The model under review builds one solid part; all positions refer to its coordinate system, in mm. A direction names the side the tool comes from. Round coordinates to 2 decimals unless told otherwise and drop trailing zeros.
Item 1: Machinability: for faces 4 (the face through (-21.863, -2.882, -0.063)), 5 (the face through (2.794, -1, 0)), 6 (the face through (-48.549, -0.705, -0.04)), 7 (the face through (0, 1, 0)), which of the approach directions +Z, -Z, +X, -X, +Y, -Y give a long, thin tool a straight path to every point of the face, cutting with its end or side? Answer none if there is none.
Item 2: Draft analysis for pull direction X (two halves, no side actions). For faces 1 (the face through (-0.387, 1.841, -0.04)), 2 (the face through (-48.661, 0.744, -0.04)), 3 (the face through (-22.638, 2.882, -0.063)), state which applies: +X half, -X half, draft (parallel to the pull), parting line (faces both ways), or undercut.
Item 3: To check wall thickness, follow L1, parallel to Z at x = -10.5, y = 2.5; L2, parallel to X at y = -1.5, z = -0.15; L3, parallel to X at y = 4.5, z = 0.7. State the ranges of each line that lie inside material, in increasing order.
Item 4: Clearance check with flat-ended pins moving along their axes: pin 1 Ø3 at (x, z) = (-33.5, 1) entering from -Y; pin 2 Ø3 at (y, z) = (-3, -1.5) entering from -X; pin 3 Ø1.5 at (x, z) = (-36.5, -1) entering from +Y. State where each tip first meets the part, or that it passes through.
```python
from build123d import *

# Parameters (mm, degrees)
CHAMFER1_SIZE = 1.42875


with BuildPart() as part:
    # Sweep1: sweep along a path in Sketch1
    with BuildLine(Plane.XY) as sweep1_path:
        Line((2.794, -0.0254), (-44.45, -0.0254))
        ThreePointArc((-44.45, -0.0254), (-48.605420273, -0.724463272), (-52.303375713, -2.744694118))
        ThreePointArc((-52.303375713, -2.744694118), (-57.955554034, 0), (-52.303375713, 2.744694118))
        ThreePointArc((-52.303375713, 2.744694118), (-48.605420273, 0.724463272), (-44.45, 0.0254))
        Line((-44.45, 0.0254), (0, 0.0254))
    # Sketch2 → Sweep1 (sweep)
    with BuildSketch(Plane(origin=(0, 0, 0), x_dir=(0, 0, -1), z_dir=(1, 0, 0))):
        with BuildLine():
            Line((-2.8575, 0.0254), (2.8575, 0.0254))
            ThreePointArc((2.8575, 0.0254), (0, 2.8829), (-2.8575, 0.0254))
        make_face()
    sweep(path=sweep1_path.line)

    # Chamfer1
    chamfer1_edges = [part.edges().sort_by_distance(p)[0] for p in [
        (2.794, -2.8829, 0),
        (0, 2.8829, 0),
    ]]
    chamfer(chamfer1_edges, length=CHAMFER1_SIZE)


solid = part.part
```
Numbers:
1. face 4: +X, -Y
1. face 5: +Z, -Z, +X, +Y, -Y
1. face 6: +Z, -Z
1. face 7: +Z, -Z, +X, +Y
2. face 1: +X half
2. face 2: undercut
2. face 3: draft
3. L1: z = -1.43 to 1.43
3. L2: x = -60.63 to -57.62, -50.39 to 2.74
3. L3: x = -58.82 to -50.01
4. pin 1: stops at y = -2.88
4. pin 2: stops at x = -60.49
4. pin 3: stops at y = 2.87
